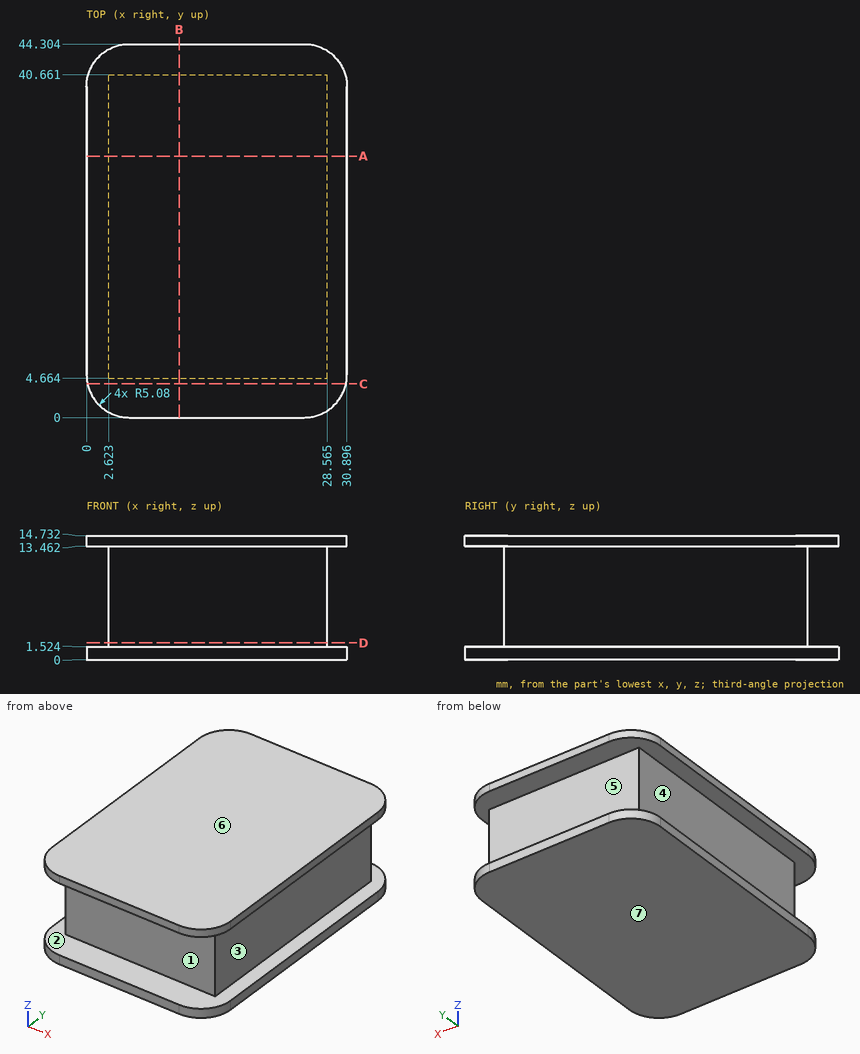
Job drawing, mm, ordinate dimensions from the low corner. One solid piece. A direction names the side the tool comes from. Coordinates: 2 decimals unless noted, no trailing zeros. Write each loop counter-clockwise with the first axis right and the second up, starting at its lowest first coordinate (ties: lowest second). Pieces come first, ordered by that corner, then holes.
Item 1: Slice it at D-D (z = 2). Write the cut outline in (x, y) (1 decimal).
Item 2: Slice it at B-B (x = 11). Write the cut outline in (y, z) (1 decimal).
Item 3: Slice it at C-C (y = 4). Write the cut outline in (x, z).
Item 4: Mould opens along Z. For the marked faces 5, 6 and 7 say: released by +Z, released by -Z, zero draft, split by the parting line, or undercut.
Item 5: Slice it at A-A (y = 31). Write the cut outline in (x, z) (1 decimal).
Item 6: Pin check, flat tips, straight feed: pin 1 (8 mm diameter, centred on x = 19, z = 7, fed in from +Y); pin 2 (2 mm diameter, centred on y = 29.5, z = 6.5, fed in from +X) (1 decimal); pin 3 (3.5 mm diameter, centred on y = 26, z = 8, fed in from -X). Stop position of each tip, or through.
Item 7: Which spindle directions (+Z, -Z, +X, -X, +Y, -Y) get a long thin tool onto all of the face, cutting with end or side? Do the marked faces 1, 2, 3 and 4. Say none if no direction does.
Item 8: Probe line 1 (Z direction, x = 17, y = 4); line 2 (Y direction, x = 18, z = 3); line 3 (X direction, y = 31, z = 11.5) (1 decimal). List the from-to ranges inside material, lowest first.
Results found:
1. outline: (2.6, 4.7) - (28.6, 4.7) - (28.6, 40.7) - (2.6, 40.7) - close
2. outline: (0, 0) - (44.3, 0) - (44.3, 1.5) - (40.7, 1.5) - (40.7, 13.5) - (44.3, 13.5) - (44.3, 14.7) - (0, 14.7) - (0, 13.5) - (4.7, 13.5) - (4.7, 1.5) - (0, 1.5) - close
3. outline: (0.12, 0) - (30.78, 0) - (30.78, 1.52) - (0.12, 1.52) - close; (0.12, 13.46) - (30.78, 13.46) - (30.78, 14.73) - (0.12, 14.73) - close
4. face 5: undercut
4. face 6: released by +Z
4. face 7: released by -Z
5. outline: (0, 0) - (30.9, 0) - (30.9, 1.5) - (28.6, 1.5) - (28.6, 13.5) - (30.9, 13.5) - (30.9, 14.7) - (0, 14.7) - (0, 13.5) - (2.6, 13.5) - (2.6, 1.5) - (0, 1.5) - close
6. pin 1: stops at y = 40.66
6. pin 2: stops at x = 28.6
6. pin 3: stops at x = 2.62
7. face 1: +X, -X, -Y
7. face 2: none
7. face 3: +X, +Y, -Y
7. face 4: -X, +Y, -Y
8. line 1: z = 0 to 1.52, 13.46 to 14.73
8. line 2: y = 4.66 to 40.66
8. line 3: x = 2.6 to 28.6
